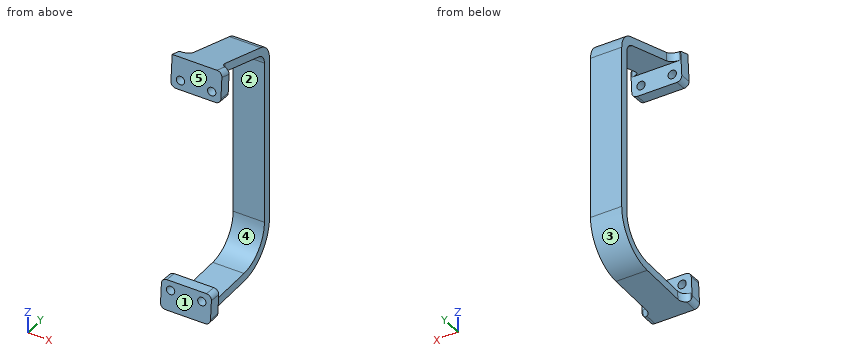
```python
from build123d import *

# Parameters (mm, degrees)
BOSS_EXTRUDE1_DEPTH = 7.5
BOSS_EXTRUDE3_DEPTH = 12
FILLET1_R           = 2.5
FILLET2_R           = 4
CUT_EXTRUDE1_REACH  = 333.875
SKETCH5_R           = 2.0000000000001186
SKETCH5_R_2         = 2.0000000000001266
SKETCH5_R_3         = 2.0000000000001346


with BuildPart() as part:
    # Sketch1 → Boss-Extrude1 (new, symmetric)
    with BuildSketch(Plane(origin=(249.7714193313032, 90.19789758644944, 68.85838392138058), x_dir=(-1.36e-15, 0, -1), z_dir=(1, 1.23e-15, -1.36e-15))):
        with BuildLine():
            Line((276.40733700705005, 27.058032303601674), (280.40733700705005, 26.750876980739832))
            Line((280.40733700705005, 26.750876980739832), (280.40733700705005, 54.805859741005065))
            ThreePointArc((280.40733700705005, 54.80585974100506), (274.549472630781, 68.947995364736), (260.40733700705005, 74.80585974100505))
            Line((260.40733700705005, 74.80585974100507), (180.40733700705002, 74.80585974100505))
            ThreePointArc((180.40733700705002, 74.80585974100504), (174.52666621732683, 72.89398134388023), (170.89462091629855, 67.88940195358433))
            Line((170.89462091629855, 67.88940195358433), (158.7191888589005, 30.328239997775782))
            Line((158.7191888589005, 30.32823999777578), (162.8219643315265, 30.01319266654476))
            Line((162.8219643315265, 30.013192666544757), (174.69970735259915, 66.65598506855262))
            ThreePointArc((174.69970735259915, 66.65598506855262), (176.8789345332161, 69.65873270273018), (180.40733700705002, 70.80585974100507))
            Line((180.40733700705002, 70.80585974100505), (260.40733700705005, 70.80585974100507))
            ThreePointArc((260.40733700705005, 70.80585974100507), (271.7210455060348, 66.1195682399898), (276.40733700705005, 54.80585974100506))
            Line((276.40733700705005, 54.80585974100506), (276.40733700705005, 27.058032303601674))
        make_face()
    extrude(amount=BOSS_EXTRUDE1_DEPTH, both=True)

    # Sketch1<4> → Boss-Extrude3 (add, symmetric)
    with BuildSketch(Plane(origin=(249.7714193313032, 90.19789758644944, 68.85838392138058), x_dir=(-1.36e-15, 0, -1), z_dir=(1, 1.23e-15, -1.36e-15))):
        Polygon((174.61655820891, 34.87442718512688), (164.64591108515557, 35.64006151923646), (162.8219643315265, 30.01319266654476), (174.17631846679706, 29.14130508896809), align=None)
        Polygon((164.64591108515557, 35.64006151923646), (160.5431356125297, 35.95510885046747), (158.7191888589005, 30.328239997775782), (162.8219643315265, 30.01319266654476), align=None)
        Polygon((276.40733700705005, 21.291104712411546), (280.40733700705005, 20.983949389549675), (280.40733700705005, 26.750876980739832), (276.40733700705005, 27.058032303601674), align=None)
        Polygon((265.9964501411826, 22.090544541552422), (276.40733700705005, 21.291104712411546), (276.40733700705005, 27.058032303601674), (266.4366898832956, 27.823666637711245), align=None)
    extrude(amount=BOSS_EXTRUDE3_DEPTH, both=True)

    # Fillet1
    fillet1_edges = [part.edges().sort_by_distance(p)[0] for p in [
        (237.77141933130292, 122.20576372349691, -105.53805441647292),
        (261.7714193313029, 122.20576372349694, -105.53805441647295),
        (261.7714193313029, 123.33957201057109, -90.77277831433453),
        (261.7714193313028, 115.1550031760813, -197.35818609085857),
        (237.7714193313028, 114.06531077159418, -211.54895308566944),
        (261.7714193313028, 114.06531077159421, -211.5489530856695),
        (237.7714193313028, 115.15500317608127, -197.3581860908585),
    ]]
    fillet(fillet1_edges, radius=FILLET1_R)

    # Fillet2
    fillet2_edges = [part.edges().sort_by_distance(p)[0] for p in [
        (257.271419331303, 125.9954827713014, -93.73613942746209),
        (242.27141933130298, 125.99548277130137, -93.73613942746206),
        (242.2714193313028, 117.10235222862019, -209.54895308566944),
        (257.2714193313028, 117.10235222862022, -209.5489530856695),
    ]]
    fillet(fillet2_edges, radius=FILLET2_R)

    # Sketch5 → Cut-Extrude1 (cut, up to next)
    with BuildSketch(Plane(origin=(-1.7714e-13, 132.41259718729538, -10.16780851001), x_dir=(1, 1.33e-15, -1e-16), z_dir=(-1.3338661735596055e-15, 0.9970647123754437, -0.07656343341095512)), mode=Mode.PRIVATE) as cut_extrude1_sk1:
        with Locations(Location((242.271419331303, 192.46222063201034, 0), (0, 0, 270))):
            Circle(SKETCH5_R)
    cut_extrude1_tool1 = extrude(cut_extrude1_sk1.sketch, amount=-CUT_EXTRUDE1_REACH, mode=Mode.PRIVATE) & part.part
    # Sketch5 → Cut-Extrude1 (cut, up to next)
    with BuildSketch(Plane(origin=(-1.7714e-13, 132.41259718729538, -10.16780851001), x_dir=(1, 1.33e-15, -1e-16), z_dir=(-1.3338661735596055e-15, 0.9970647123754437, -0.07656343341095512)), mode=Mode.PRIVATE) as cut_extrude1_sk2:
        with Locations(Location((257.2714193313028, 192.46222063201034, 0), (0, 0, 270))):
            Circle(SKETCH5_R_2)
    cut_extrude1_tool2 = extrude(cut_extrude1_sk2.sketch, amount=-CUT_EXTRUDE1_REACH, mode=Mode.PRIVATE) & part.part
    # Sketch5 → Cut-Extrude1 (cut, up to next)
    with BuildSketch(Plane(origin=(-1.7714e-13, 132.41259718729538, -10.16780851001), x_dir=(1, 1.33e-15, -1e-16), z_dir=(-1.3338661735596055e-15, 0.9970647123754437, -0.07656343341095512)), mode=Mode.PRIVATE) as cut_extrude1_sk3:
        with Locations(Location((242.27141933130304, 91.37177701814517, 0), (0, 0, 270))):
            Circle(SKETCH5_R_3)
    cut_extrude1_tool3 = extrude(cut_extrude1_sk3.sketch, amount=-CUT_EXTRUDE1_REACH, mode=Mode.PRIVATE) & part.part
    # Sketch5 → Cut-Extrude1 (cut, up to next)
    with BuildSketch(Plane(origin=(-1.7714e-13, 132.41259718729538, -10.16780851001), x_dir=(1, 1.33e-15, -1e-16), z_dir=(-1.3338661735596055e-15, 0.9970647123754437, -0.07656343341095512)), mode=Mode.PRIVATE) as cut_extrude1_sk4:
        with Locations(Location((257.27141933130287, 91.37177701814517, 0), (0, 0, 270))):
            Circle(SKETCH5_R_3)
    cut_extrude1_tool4 = extrude(cut_extrude1_sk4.sketch, amount=-CUT_EXTRUDE1_REACH, mode=Mode.PRIVATE) & part.part
    add(cut_extrude1_tool1.solids().sort_by_distance((242.271419, 117.677029, -202.065097))[0], mode=Mode.SUBTRACT)
    add(cut_extrude1_tool2.solids().sort_by_distance((257.271419, 117.677029, -202.065097))[0], mode=Mode.SUBTRACT)
    add(cut_extrude1_tool3.solids().sort_by_distance((242.271419, 125.41686, -101.271383))[0], mode=Mode.SUBTRACT)
    add(cut_extrude1_tool4.solids().sort_by_distance((257.271419, 125.41686, -101.271383))[0], mode=Mode.SUBTRACT)


solid = part.part
```
Geometry check sheet. Reference: the model listing, model coordinates, mm. Face numbers are marked on the shaded views. A direction names the side the tool comes from. Coordinates: 2 decimals unless noted, no trailing zeros. Loops run counter-clockwise (first coordinate to the right, second up) from the corner with the lowest first, then second, coordinate; pieces in that order, holes last. Notation, with made-up numbers: (8, 62) -> (49, 62) arc R21 ccw to (49, 70) -> close; hole circle Ø10 at (34, 77.5). An arc over 180 degrees is marked (long way). Put each result on its own line as item: value.
1) Cross-section at C-C on z = -201.5. Count the separate pieces of the cut face and the enclosed holes in it, plus the area to 3 significant figures.
Result set:
separate pieces: 4
enclosed holes: 0
area: 165 mm^2
2) Gauge pin test, flat ends, axial feed: pin 1 Ø1 at (x, y) = (248, 150.5) entering from -Z; pin 2 Ø8 at (x, z) = (250.5, -106.5) entering from -Y; pin 3 Ø5 at (x, z) = (240.5, -172.5) entering from -Y. Record the tip position at first contact, or that the pin passes through.
Result set:
pin 1: stops at z = -210.91
pin 2: stops at y = 119.34
pin 3: stops at y = 161
3) Thickness scan on line 1 (Y direction, x = 243.75, z = -120); line 2 (Z direction, x = 256.5, y = 131); line 3 (Z direction, x = 253, y = 137.5). Record the ranges inside material, lowest first.
Result set:
line 1: y = 161 to 165
line 2: z = -211.55 to -207.55, -97.46 to -93.26
line 3: z = -211.55 to -207.55, -99.57 to -95.36
4) Release check for a two-part mould opening along Z. For the marked faces 3, 4 and 5 record: released by +Z, released by -Z, zero draft, split by the parting line, or undercut.
Result set:
face 3: released by -Z
face 4: undercut
face 5: released by +Z
5) Tool access check on the marked faces 1 and 2. Record the directions out of +Z, -Z, +X, -X, +Y, -Y that give a thin tool (end or side, any length) a straight path to the whole face; none if there is none.
Result set:
face 1: +Z, +X, -X, -Y
face 2: +X, -X, -Y
6) Cross-section at A-A on x = 248.75. Record the boundary of the cut face in (y, z), plus the area to 3 significant figures.
Result set:
outline: (111.18, -211.55) -> (145, -211.55) arc R20 ccw to (165, -191.55) -> (165, -111.55) arc R10 ccw to (158.09, -102.04) -> (120.53, -89.86) -> (119.34, -105.32) -> (125.07, -105.76) -> (125.84, -95.79) -> (156.85, -105.84) arc R6 cw to (161, -111.55) -> (161, -191.55) arc R16 cw to (145, -207.55) -> (117.26, -207.55) -> (118.02, -197.58) -> (112.29, -197.14) -> close
area: 884 mm^2
7) Cross-section at D-D on y = 136. Record the boundary of the cut face in (x, z).
Result set:
outline: (242.27, -211.55) -> (257.27, -211.55) -> (257.27, -207.55) -> (242.27, -207.55) -> close; (242.27, -99.08) -> (257.27, -99.08) -> (257.27, -94.88) -> (242.27, -94.88) -> close
8) Cross-section at B-B on y = 153. Record the boundary of the cut face in (x, z).
Result set:
outline: (242.27, -209.88) -> (257.27, -209.88) -> (257.27, -205.41) -> (242.27, -205.41) -> close; (242.27, -104.59) -> (257.27, -104.59) -> (257.27, -100.39) -> (242.27, -100.39) -> close
